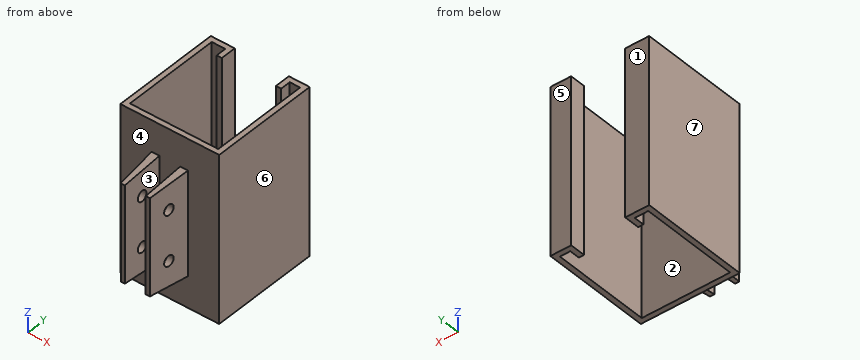
from build123d import *

# Parameters (mm, degrees)
BOSS_EXTRUDE1_DEPTH     = 101.6
SKETCH2_W               = 22.225
SKETCH2_H               = 63.5
BOSS_EXTRUDE2_DEPTH     = 25.4
BOSS_EXTRUDE2_TAPER     = 5
SKETCH2_3_W             = 12.7
SKETCH2_3_H             = 63.5
CUT_EXTRUDE1_DEPTH      = 25.4
CUT_EXTRUDE2_DEPTH      = 140.85325407
CUT_EXTRUDE2_DEPTH_BACK = 140.85325407
SKETCH3_R               = 3.175


with BuildPart() as part:
    # Sketch1 → Boss-Extrude1 (new body)
    with BuildSketch(Plane.XY):
        Polygon((0, 0), (0, -60.325), (53.975, -60.325), (53.975, 0), (47.625, 0), (47.625, -6.35), (44.45, -6.35), (44.45, 3.175), (57.15, 3.175), (57.15, -63.5), (-3.175, -63.5), (-3.175, 3.175), (11.43, 3.175), (11.43, -6.35), (8.255, -6.35), (8.255, 0), align=None)
    extrude(amount=BOSS_EXTRUDE1_DEPTH)

    # Sketch2 → Boss-Extrude2 (add)
    with BuildSketch(Plane(origin=(0, -63.5, 0), x_dir=(-1, 0, 0), z_dir=(0, -1, 0))):
        with Locations((-26.9875, -50.8)):
            Rectangle(SKETCH2_W, SKETCH2_H)
    extrude(amount=BOSS_EXTRUDE2_DEPTH, taper=BOSS_EXTRUDE2_TAPER)

    # Sketch2<3> → Cut-Extrude1 (cut)
    with BuildSketch(Plane(origin=(0, -63.5, 0), x_dir=(-1, 0, 0), z_dir=(0, -1, 0))):
        with Locations((-26.9875, -50.8)):
            Rectangle(SKETCH2_3_W, SKETCH2_3_H)
    extrude(amount=CUT_EXTRUDE1_DEPTH, mode=Mode.SUBTRACT)

    # Sketch3 → Cut-Extrude2 (cut, two sides: drawn at the far end of the back side and taken through both)
    with BuildSketch(Plane(origin=(20.6375, 0, 0), x_dir=(0, 0, -1), z_dir=(1, 0, 0)).offset(-CUT_EXTRUDE2_DEPTH_BACK)):
        with Locations(Location((-66.119446987, -76.2, 0), (0, 0, 270))):
            Circle(SKETCH3_R)
        with Locations(Location((-35.480553013, -76.2, 0), (0, 0, 270))):
            Circle(SKETCH3_R)
    extrude(amount=CUT_EXTRUDE2_DEPTH + CUT_EXTRUDE2_DEPTH_BACK, mode=Mode.SUBTRACT)


solid = part.part
Geometry: final body of the model. Coordinates: model frame, mm. Face numbers are marked on the shaded views. A direction names the side the tool comes from. Round coordinates to 2 decimals unless told otherwise and drop trailing zeros. Order: outer loops, then holes, each group sorted by start corner. A loop starts at its lowest first (then second) coordinate and runs counter-clockwise, first axis right, second up.
Q1. Pin query (flat end, axial travel): pin 1 (5 mm diameter, centred on x = 9.5, z = 81, fed in from -Y); pin 2 (8.5 mm diameter, centred on y = -76.2, z = 66.12, fed in from +X); pin 3 (10 mm diameter, centred on x = 23.5, z = 11.5, fed in from +Y) (3 decimals); pin 4 (4 mm diameter, centred on y = -76.2, z = 35.48, fed in from +X). Return the tip coordinate at first contact, or that it passes through.
Result sheet:
pin 1: stops at y = -63.5
pin 2: stops at x = 37.36
pin 3: stops at y = -60.325
pin 4: passes through
Q2. Section A-A, the plane y = -50.5. Output: boundary loops of the cut face in (x, z) (3 decimals), and give its area (3 significant figures).
Result sheet:
outline: (-3.175, 0) - (0, 0) - (0, 101.6) - (-3.175, 101.6) - close; (53.975, 0) - (57.15, 0) - (57.15, 101.6) - (53.975, 101.6) - close
area: 645 mm2
Q3. Material intervals for probe 1 along X at (y, z) = (-43.5, 25) (3 decimals); probe 2 along Y at (x, z) = (4, 37) (3 decimals); probe 3 along Z at (x, y) = (34.8, -76.2), sorted ascending.
Result sheet:
probe 1: x = -3.175 to 0, 53.975 to 57.15
probe 2: y = -63.5 to -60.325, 0 to 3.175
probe 3: z = 20.16 to 32.31, 38.66 to 62.94, 69.29 to 81.44
Q4. Section C-C, the plane z = 17.5. Output: boundary loops of the cut face in (x, y) (3 decimals).
Result sheet:
outline: (-3.175, -63.5) - (57.15, -63.5) - (57.15, 3.175) - (44.45, 3.175) - (44.45, -6.35) - (47.625, -6.35) - (47.625, 0) - (53.975, 0) - (53.975, -60.325) - (0, -60.325) - (0, 0) - (8.255, 0) - (8.255, -6.35) - (11.43, -6.35) - (11.43, 3.175) - (-3.175, 3.175) - close
Q5. Section D-D, the plane y = -76.2. Give the number of separate pieces and of enclosed holes in the cut face, and give its area (3 significant figures).
Result sheet:
separate pieces: 6
enclosed holes: 0
area: 355 mm2
Q6. Section B-B, the plane x = 49.5. Output: boundary loops of the cut face in (y, z) (3 decimals), and give its area (3 significant figures).
Result sheet:
outline: (-63.5, 0) - (-60.325, 0) - (-60.325, 101.6) - (-63.5, 101.6) - close; (0, 0) - (3.175, 0) - (3.175, 101.6) - (0, 101.6) - close
area: 645 mm2
Q7. Mould query, pull axis X, two halves, no side actions, for the marked faces 4, 5, 6 and 7. Classes: released by +X, released by -X, zero draft, split by the parting line, or undercut.
Result sheet:
face 4: undercut
face 5: zero draft
face 6: released by +X
face 7: released by -X
Q8. Access query for the marked faces 1, 2 and 3. Directions: +Z, -Z, +X, -X, +Y, -Y. A direction counts if a zero-diameter tool reaches every point of the face in a straight line with its end or side. Return the directions, or none.
Result sheet:
face 1: +Z, -Z, +X, -X, +Y
face 2: +Z, -Z
face 3: +Z, -Z, -Y
